```python
from build123d import *

# Parameters (mm, degrees)
SKETCH_1_R          = 1.2
EXTRUDE_1_DEPTH     = 2
SKETCH_2_W          = 5.828282036
SKETCH_2_H          = 6
EXTRUDE_3_DEPTH     = 6
SKETCH_4_R          = 1.5
CUT_EXTRUDE_1_DEPTH = 5.828282036
EXTRUDE_4_DEPTH     = 45
EXTRUDE_5_DEPTH     = 52.422321


with BuildPart() as part:
    # 草图1 → 凸台-拉伸1 (new body)
    # profile 1 of 3: a face of its own
    with BuildSketch(Plane.XY):
        Polygon((-105.285311989, -8.55), (-141.174369577, -8.55), (-145.174369577, -14.55), (-161.297950566, -14.55), (-164.165207203, -8.55), (-165.3, -8.55), (-165.3, -4.7), (-168, -4.7), (-168, 65), (-165.3, 65), (-159.471717964, 65), (-149.4421323, 68.256733276), (-149.4421323, 63.85), (-141.4421323, 63.85), (-141.4421323, 68.85), (-104.45, 68.85), (-104.45, 60.3), (-117.895945033, 50.15), (-117.895945033, 10.15), (-105.285311989, 0), align=None)
    # profile 2 of 3: a face of its own
    with BuildSketch(Plane.XY):
        Polygon((-141.4421323, 63.85), (-141.4421323, 68.85), (-104.45, 68.85), (-104.45, 60.3), (-95.7, 60.3), (-104.45, 70.65), (-147.9, 70.65), (-165.3, 65), (-159.471717964, 65), (-149.4421323, 68.256733276), (-149.4421323, 63.85), align=None)
        with Locations((-101.45, 63.5)):
            Circle(SKETCH_1_R, mode=Mode.SUBTRACT)
        with Locations((-145.6421323, 67.45)):
            Circle(SKETCH_1_R, mode=Mode.SUBTRACT)
    # profile 3 of 3: a face of its own
    with BuildSketch(Plane.XY):
        Polygon((-105.285311989, 0), (-105.285311989, -8.55), (-141.174369577, -8.55), (-145.174369577, -14.55), (-161.297950566, -14.55), (-164.165207203, -8.55), (-165.3, -8.55), (-165.3, -4.7), (-168, -4.7), (-162.432743363, -16.35), (-141.174369577, -16.35), (-137.174369577, -10.35), (-104.45, -10.35), (-95.7, 0), align=None)
        with Locations((-140.974369577, -12.15)):
            Circle(SKETCH_1_R, mode=Mode.SUBTRACT)
        with Locations((-102.285311989, -3.2)):
            Circle(SKETCH_1_R, mode=Mode.SUBTRACT)
    extrude(amount=EXTRUDE_1_DEPTH)

    # 草图2 → 凸台-拉伸3 (add)
    with BuildSketch(Plane(origin=(0, 0, 0), x_dir=(-1, 0, 0), z_dir=(0, 0, -1))):
        with Locations((162.385858982, 62)):
            Rectangle(SKETCH_2_W, SKETCH_2_H)
        with Locations((162.385858982, -1.7)):
            Rectangle(SKETCH_2_W, SKETCH_2_H)
    extrude(amount=EXTRUDE_3_DEPTH)

    # 草图4 → 切除-拉伸1 (cut)
    with BuildSketch(Plane.ZY.offset(165.3)):
        with Locations(Location((-3.1, 61.9, 0), (0, 0, 270))):
            Circle(SKETCH_4_R)
        with Locations(Location((-3.1, -1.6, 0), (0, 0, 270))):
            Circle(SKETCH_4_R)
    extrude(amount=-CUT_EXTRUDE_1_DEPTH, mode=Mode.SUBTRACT)

    # 草图5 → 凸台-拉伸4 (add)
    with BuildSketch(Plane.XY.offset(2)):
        Polygon((-113, 54.9), (-168, 54.9), (-168, 51.9), (-115.577678648, 51.9), (-111.603507702, 54.9), align=None)
        Polygon((-115.721697956, 8.4), (-168, 8.4), (-168, 5.4), (-113, 5.4), (-111.994417254, 5.4), align=None)
    extrude(amount=EXTRUDE_4_DEPTH)

    # 草图6 → 凸台-拉伸5 (add)
    with BuildSketch(Plane.ZY.offset(168)):
        Polygon((47, 54.9), (47, 52.65), (55, 52.65), (57, 52.65), (57, 54.9), align=None)
        Polygon((55, 7.65), (47, 7.65), (47, 5.4), (57, 5.4), (57, 8.4), (55, 8.4), align=None)
    extrude(amount=-EXTRUDE_5_DEPTH)


solid = part.part
```
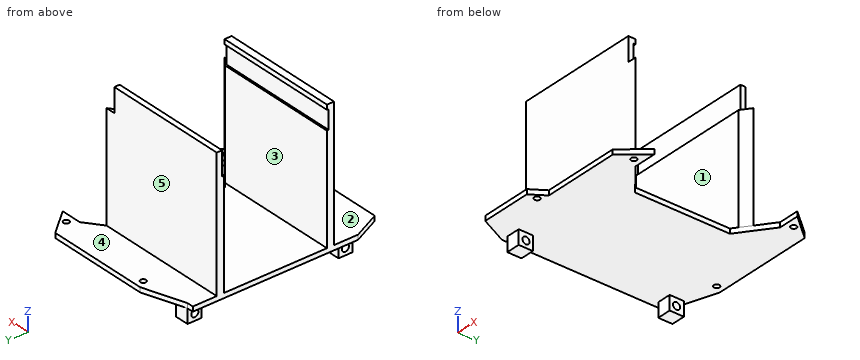
For this review, take the finished solid that the model builds, in its own axes (mm). Face numbers are marked on the shaded views. A direction names the side the tool comes from. Round coordinates to 2 decimals unless told otherwise and drop trailing zeros. Order: outer loops, then holes, each group sorted by start corner. A loop starts at its lowest first (then second) coordinate and runs counter-clockwise, first axis right, second up. Notation, with made-up numbers: (-38.75, 59.25) -> (-2.75, 59.25) arc R14 cw to (-2.75, 64.25) -> close; hole circle Ø6 at (39.5, 60.25). An arc over 180 degrees is marked (long way). Use a Markdown table: item, result.
Item 1: Take a section at C-C (x = -109.5). State the section outline as (y, z) points.
Resolved:
| item | result |
|---|---|
| outline | (-10.35, 0) -> (3.39, 0) -> (3.39, 2) -> (-10.35, 2) -> close; (56.49, 0) -> (70.65, 0) -> (70.65, 2) -> (56.49, 2) -> close |
Item 2: Take a section at A-A (z = -3.1). State the section outline as (x, y) points.
Resolved:
| item | result |
|---|---|
| outline | (-165.3, -4.7) -> (-159.47, -4.7) -> (-159.47, -3.1) -> (-165.3, -3.1) -> close; (-165.3, -0.1) -> (-159.47, -0.1) -> (-159.47, 1.3) -> (-165.3, 1.3) -> close; (-165.3, 59) -> (-159.47, 59) -> (-159.47, 60.4) -> (-165.3, 60.4) -> close; (-165.3, 63.4) -> (-159.47, 63.4) -> (-159.47, 65) -> (-165.3, 65) -> close |
Item 3: For line 1 along Y through (x, z) = (-164.5, 50.5); line 2 along Y through (x, z) = (-130, 16); line 3 along Z through (x, y) = (-162.9, -1.6), list the stretches that pass through material, from the lowest coordinate up. Write a range as [from, to].
Resolved:
| item | result |
|---|---|
| line 1 | y = [5.4, 7.65], [52.65, 54.9] |
| line 2 | y = [5.4, 8.4], [51.9, 54.9] |
| line 3 | z = [-6, -4.6], [-1.6, 2] |
Item 4: Take a section at D-D (x = -134.5). State the section outline as (y, z) points, plus the area to 4 significant figures.
Resolved:
| item | result |
|---|---|
| outline | (-10.35, 0) -> (70.65, 0) -> (70.65, 2) -> (54.9, 2) -> (54.9, 57) -> (52.65, 57) -> (52.65, 47) -> (51.9, 47) -> (51.9, 2) -> (8.4, 2) -> (8.4, 47) -> (7.65, 47) -> (7.65, 55) -> (8.4, 55) -> (8.4, 57) -> (5.4, 57) -> (5.4, 2) -> (-10.35, 2) -> close |
| area | 478.5 mm² |
Item 5: For pin 1 (1.8 mm diameter, centred on y = -1.5, z = -1.5, fed in from +X); pin 2 (2 mm diameter, centred on x = -137, y = 48.5, fed in from -Z); pin 3 (1.8 mm diameter, centred on y = 61.9, z = -3.1, fed in from -X); pin 4 (2 mm diameter, centred on x = -127, z = 46, fed in from -Y), all flat-tipped, find the tip position at first contact; note any pin that passes through.
Resolved:
| item | result |
|---|---|
| pin 1 | stops at x = -159.47 |
| pin 2 | stops at z = 0 |
| pin 3 | passes through |
| pin 4 | stops at y = 5.4 |
Item 6: Machinability: for the marked faces 1 and 2, which of the approach directions +Z, -Z, +X, -X, +Y, -Y give a long, thin tool a straight path to every point of the face, cutting with its end or side? Answer none if there is none.
Resolved:
| item | result |
|---|---|
| face 1 | +Z, +X, -X |
| face 2 | +Z, +X, -X, -Y |
Item 7: Take a section at B-B (z = 32). State the section outline as (x, y) points, plus the area to 3 significant figures.
Resolved:
| item | result |
|---|---|
| outline | (-168, 5.4) -> (-111.99, 5.4) -> (-115.72, 8.4) -> (-168, 8.4) -> close; (-168, 51.9) -> (-115.58, 51.9) -> (-111.6, 54.9) -> (-168, 54.9) -> close |
| area | 326 mm² |
Item 8: Draft analysis for pull direction Y (two halves, no side actions). For the marked faces 3, 4 and 5, state which applies: +Y half, -Y half, draft (parallel to the pull), parting line (faces both ways), or undercut.
Resolved:
| item | result |
|---|---|
| face 3 | undercut |
| face 4 | draft |
| face 5 | +Y half |
